The model under review builds one solid part; all positions refer to its coordinate system, in mm. A direction names the side the tool comes from. Coordinates: 2 decimals unless noted, no trailing zeros. Order: outer loops, then holes, each group sorted by start corner. A loop starts at its lowest first (then second) coordinate and runs counter-clockwise, first axis right, second up. Notation, with made-up numbers: (38.5, 32.25) -> (45.5, 32.25) arc R19 cw to (45.5, 48.25) -> close; hole circle Ø4 at (47.5, -9.5). An arc over 180 degrees is marked (long way). Use one line per item in the form item = value. Start each with the question number.
(1) Take a section at B-B (x = -20.5). State the section outline as (y, z) points.
(2) For faces 4 (the flat face through (4.155, 22, -24)), 5 (the flat face through (4, 49, -24)), 6 (the flat face through (-35, 49, 13)), 7 (the flat face through (50.799, 27, -10)), list the 3-axis set-ups (+Z, -Z, +X, -X, +Y, -Y) from which the entire face can be reached by the end or side of a thin tool; tool diameter is ignored.
(3) Take a section at C-C (y = 8.5). State the section outline as (x, z) points.
(4) Mouldability with a two-part tool opening along X and no side actions: class faces 1 (the flat face through (-35, 49, -7)), 2 (the flat face through (17, 27, -22.84)), 3 (the flat face through (26.149, 51, -24)) as +X half, -X half, draft (parallel to the pull), parting line (faces both ways), or undercut.
(5) Wall thickness on line 1 along X through (y, z) = (27.5, -21); line 2 along X through (y, z) = (43.5, 14); line 3 along Z through (x, y) = (30, 4.5): over which ranges is each line inside the solid? List them lowest first.
(6) Take a section at D-D (z = -8). State the section outline as (x, y) points.
(7) Take a section at A-A (y = 18.5). State the section outline as (x, z) points, then the cut area to 3 significant figures.
(8) Insertion check: pin 1 Ø1.5 at (x, z) = (28, 26) entering from +Y; pin 2 Ø2.5 at (y, z) = (14.5, -23.5) entering from +X; pin 3 Ø12 at (x, y) = (39, 43) entering from +Z. Each pin has a flat end and moves straight along its axis. Give the tip position at first contact, or say it passes through.
```python
from build123d import *

# Parameters (mm, degrees)
SKETCH1_W           = 90.3
SKETCH1_H           = 58.17
BOSS_EXTRUDE1_DEPTH = 2
SKETCH4_W           = 28.4
SKETCH4_H           = 32.2
BOSS_EXTRUDE2_DEPTH = 2
BOSS_EXTRUDE3_DEPTH = 20
SKETCH6_W           = 3
SKETCH6_H           = 58.17
BOSS_EXTRUDE4_DEPTH = 50
SKETCH7_W           = 15.3
SKETCH7_H           = 4
CUT_EXTRUDE1_DEPTH  = 4
SKETCH8_W           = 10
SKETCH8_H           = 3
SKETCH8_W_2         = 22
BOSS_EXTRUDE5_DEPTH = 50
SKETCH9_W           = 3
SKETCH9_H           = 9
BOSS_EXTRUDE7_DEPTH = 30
BOSS_EXTRUDE8_DEPTH = 30
SKETCH11_W          = 2
SKETCH11_H          = 3
BOSS_EXTRUDE9_DEPTH = 50
SKETCH12_W          = 10
SKETCH12_H          = 26
CUT_EXTRUDE2_DEPTH  = 5
SKETCH13_W          = 3
SKETCH13_H          = 5
SKETCH13_W_2        = 5
SKETCH13_H_2        = 3
SKETCH13_W_3        = 32.5
SKETCH13_H_3        = 32.2
CUT_EXTRUDE3_DEPTH  = 3


with BuildPart() as part:
    # Sketch1 → Boss-Extrude1 (new body)
    with BuildSketch(Plane(origin=(0, 0, 0), x_dir=(1, 0, 0), z_dir=(0, 1, 0))):
        with Locations((8.649006711, -3.245187919)):
            Rectangle(SKETCH1_W, SKETCH1_H)
    extrude(amount=BOSS_EXTRUDE1_DEPTH)

    # Sketch4 → Boss-Extrude2 (add)
    with BuildSketch(Plane(origin=(0, 2, 0), x_dir=(1, 0, 0), z_dir=(0, 1, 0))):
        with Locations((67.999006711, -16.230187919)):
            Rectangle(SKETCH4_W, SKETCH4_H)
    extrude(amount=-BOSS_EXTRUDE2_DEPTH)

    # Sketch5 → Boss-Extrude3 (add)
    with BuildSketch(Plane(origin=(0, 2, 0), x_dir=(1, 0, 0), z_dir=(0, 1, 0))):
        Polygon((82.199006711, -0.130187919), (82.199006711, -32.330187919), (49.699006711, -32.330187919), (49.699006711, -29.330187919), (79.199006711, -29.330187919), (79.199006711, -3.130187919), (50.799006711, -3.130187919), (50.799006711, 22.839812081), (26.155250354, 22.839812081), (26.155250354, 25.839812081), (53.799006711, 25.839812081), (53.799006711, -0.130187919), align=None)
    extrude(amount=BOSS_EXTRUDE3_DEPTH)

    # Sketch6 → Boss-Extrude4 (add)
    with BuildSketch(Plane(origin=(0, 2, 0), x_dir=(1, 0, 0), z_dir=(0, 1, 0))):
        with Locations((-35.000993289, -3.245187919)):
            Rectangle(SKETCH6_W, SKETCH6_H)
    extrude(amount=BOSS_EXTRUDE4_DEPTH)

    # Sketch7 → Cut-Extrude1 (cut)
    with BuildSketch(Plane.ZY.offset(36.500993289)):
        with Locations((10.470187919, 8.31)):
            Rectangle(SKETCH7_W, SKETCH7_H)
    extrude(amount=-CUT_EXTRUDE1_DEPTH, mode=Mode.SUBTRACT)

    # Sketch8 → Boss-Extrude5 (add)
    with BuildSketch(Plane(origin=(0, 2, 0), x_dir=(1, 0, 0), z_dir=(0, 1, 0))):
        with Locations((-28.500993289, 24.339812081)):
            Rectangle(SKETCH8_W, SKETCH8_H)
        with Locations((15.155250354, 24.339812081)):
            Rectangle(SKETCH8_W_2, SKETCH8_H)
    extrude(amount=BOSS_EXTRUDE5_DEPTH)

    # Sketch9 → Boss-Extrude7 (add)
    with BuildSketch(Plane.ZY.offset(-4.155250354)):
        with Locations((-24.339812081, 47.5)):
            Rectangle(SKETCH9_W, SKETCH9_H)
    extrude(amount=BOSS_EXTRUDE7_DEPTH)

    # Sketch10 → Boss-Extrude8 (add)
    with BuildSketch(Plane(origin=(0, 22, 0), x_dir=(1, 0, 0), z_dir=(0, 1, 0))):
        Polygon((26.155250354, 25.839812081), (26.155250354, 22.839812081), (50.799006711, 22.839812081), (50.799006711, -3.130187919), (79.199006711, -3.130187919), (79.199006711, -29.330187919), (49.699006711, -29.330187919), (49.699006711, -32.330187919), (82.199006711, -32.330187919), (82.199006711, -0.130187919), (53.799006711, -0.130187919), (53.799006711, 25.839812081), align=None)
    extrude(amount=BOSS_EXTRUDE8_DEPTH)

    # Sketch11 → Boss-Extrude9 (add)
    with BuildSketch(Plane(origin=(0, 2, 0), x_dir=(1, 0, 0), z_dir=(0, 1, 0))):
        with Locations((-32.500993289, -30.830187919)):
            Rectangle(SKETCH11_W, SKETCH11_H)
    extrude(amount=BOSS_EXTRUDE9_DEPTH)

    # Sketch12 → Cut-Extrude2 (cut)
    with BuildSketch(Plane.XY.offset(32.330187919)):
        with Locations((54.699006711, 33)):
            Rectangle(SKETCH12_W, SKETCH12_H)
    extrude(amount=-CUT_EXTRUDE2_DEPTH, mode=Mode.SUBTRACT)

    # Sketch13 → Cut-Extrude3 (cut)
    with BuildSketch(Plane(origin=(0, 52, 0), x_dir=(1, 0, 0), z_dir=(0, 1, 0))):
        with Locations((-35.000993289, -23.245187919)):
            Rectangle(SKETCH13_W, SKETCH13_H)
        with Locations((-35.000993289, -13.245187919)):
            Rectangle(SKETCH13_W, SKETCH13_H)
        with Locations((-35.000993289, -3.245187919)):
            Rectangle(SKETCH13_W, SKETCH13_H)
        with Locations((-35.000993289, 6.754812081)):
            Rectangle(SKETCH13_W, SKETCH13_H)
        with Locations((-35.000993289, 16.754812081)):
            Rectangle(SKETCH13_W, SKETCH13_H)
        with Locations((-26.350993289, 24.339812081)):
            Rectangle(SKETCH13_W_2, SKETCH13_H_2)
        with Locations((-16.350993289, 24.339812081)):
            Rectangle(SKETCH13_W_2, SKETCH13_H_2)
        with Locations((-6.350993289, 24.339812081)):
            Rectangle(SKETCH13_W_2, SKETCH13_H_2)
        with Locations((3.649006711, 24.339812081)):
            Rectangle(SKETCH13_W_2, SKETCH13_H_2)
        with Locations((13.649006711, 24.339812081)):
            Rectangle(SKETCH13_W_2, SKETCH13_H_2)
        with Locations((23.649006711, 24.339812081)):
            Rectangle(SKETCH13_W_2, SKETCH13_H_2)
        with Locations((33.649006711, 24.339812081)):
            Rectangle(SKETCH13_W_2, SKETCH13_H_2)
        with Locations((43.649006711, 24.339812081)):
            Rectangle(SKETCH13_W_2, SKETCH13_H_2)
        with Locations((65.949006711, -16.230187919)):
            Rectangle(SKETCH13_W_3, SKETCH13_H_3)
        with Locations((52.299006711, 18.239812081)):
            Rectangle(SKETCH13_W, SKETCH13_H)
        with Locations((52.299006711, 8.239812081)):
            Rectangle(SKETCH13_W, SKETCH13_H)
    extrude(amount=-CUT_EXTRUDE3_DEPTH, mode=Mode.SUBTRACT)


solid = part.part
```
Findings:
q1.outline = (0, -25.84) -> (2, -25.84) -> (2, 32.33) -> (0, 32.33) -> close; (43, -25.84) -> (52, -25.84) -> (52, -22.84) -> (43, -22.84) -> close
q2.face_4 = +Z, -Z
q2.face_5 = +Z, -Z, +Y
q2.face_6 = +X, -X, +Y
q2.face_7 = +Y
q3.outline = (-36.5, -25.84) -> (-23.5, -25.84) -> (-23.5, -22.84) -> (-33.5, -22.84) -> (-33.5, 2.82) -> (-36.5, 2.82) -> close; (-36.5, 18.12) -> (-33.5, 18.12) -> (-33.5, 29.33) -> (-31.5, 29.33) -> (-31.5, 32.33) -> (-36.5, 32.33) -> close; (4.16, -25.84) -> (53.8, -25.84) -> (53.8, 0.13) -> (82.2, 0.13) -> (82.2, 32.33) -> (49.7, 32.33) -> (49.7, 29.33) -> (79.2, 29.33) -> (79.2, 3.13) -> (50.8, 3.13) -> (50.8, -22.84) -> (4.16, -22.84) -> close
q4.face_1 = draft
q4.face_2 = undercut
q4.face_3 = undercut
q5.line_1 = -36.5 to -33.5, 50.8 to 53.8
q5.line_2 = -36.5 to -33.5, 79.2 to 82.2
q5.line_3 = -25.84 to -22.84
q6.outline = (-36.5, 0) -> (53.8, 0) -> (53.8, 49) -> (50.8, 49) -> (50.8, 2) -> (-33.5, 2) -> (-33.5, 49) -> (-36.5, 49) -> close
q7.outline = (-36.5, -25.84) -> (-23.5, -25.84) -> (-23.5, -22.84) -> (-33.5, -22.84) -> (-33.5, 29.33) -> (-31.5, 29.33) -> (-31.5, 32.33) -> (-36.5, 32.33) -> close; (4.16, -25.84) -> (53.8, -25.84) -> (53.8, 0.13) -> (82.2, 0.13) -> (82.2, 32.33) -> (49.7, 32.33) -> (49.7, 29.33) -> (79.2, 29.33) -> (79.2, 3.13) -> (50.8, 3.13) -> (50.8, -22.84) -> (4.16, -22.84) -> close
q7.area = 699 mm²
q8.pin_1 = 2
q8.pin_2 = 53.8
q8.pin_3 = -22.84
